Part model, mm, in its own coordinate system. Face numbers are marked on the shaded views. A direction names the side the tool comes from. Coordinates: 2 decimals unless noted, no trailing zeros. Loops run counter-clockwise (first coordinate to the right, second up) from the corner with the lowest first, then second, coordinate; pieces in that order, holes last. Notation, with made-up numbers: (49, 69) - (98, 69) arc R17 cw to (98, 78) - close; hole circle Ø1 at (49, -21.75). An arc over 180 degrees is marked (long way). Answer as CSV lines item,"result".
from build123d import *

# Parameters (mm, degrees)
SKETCH1_R           = 5
BASEHEAD_DEPTH      = 6
SKETCH2_R           = 3
BASEBODY_DEPTH      = 12
HEXAGONSOCKET_DEPTH = 3
TOPFILLET_R         = 0.75
CHAMFER1_SIZE       = 0.25
LPATTERN10_COUNT    = 18
LPATTERN10_PITCH    = 0.6498


with BuildPart() as part:
    # Sketch1 → BaseHead (new body)
    with BuildSketch(Plane(origin=(0, 0, 0), x_dir=(0, 0, -1), z_dir=(1, 0, 0))):
        Circle(SKETCH1_R)
    extrude(amount=BASEHEAD_DEPTH)

    # Sketch2 → BaseBody (add)
    with BuildSketch(Plane(origin=(6, 0, 0), x_dir=(0, 0, -1), z_dir=(1, 0, 0))):
        Circle(SKETCH2_R)
    extrude(amount=BASEBODY_DEPTH)

    # Sketch3 → HexagonSocket (cut)
    with BuildSketch(Plane(origin=(0, 0, 0), x_dir=(0, 0, -1), z_dir=(1, 0, 0))):
        Polygon((2.886751346, 0), (1.443375673, 2.5), (-1.443375673, 2.5), (-2.886751346, 0), (-1.443375673, -2.5), (1.443375673, -2.5), align=None)
    extrude(amount=HEXAGONSOCKET_DEPTH, mode=Mode.SUBTRACT)

    # Sketch4 → Cut-Revolve1 (revolve, cut)
    with BuildSketch(Plane(origin=(-4.19613823, 0.75, 0), x_dir=(-1, 0, 0), z_dir=(0, 0, 1))):
        Polygon((-7.19613823, 3.25), (-8.639513903, 0.75), (-7.19613823, 0.75), align=None)
    revolve(axis=Axis((0.838992387, 0, 0), (-1, 0, 0)), mode=Mode.SUBTRACT)

    # TopFillet
    topfillet_edges = [part.edges().sort_by_distance(p)[0] for p in [
        (0, 0, 5),
    ]]
    fillet(topfillet_edges, radius=TOPFILLET_R)

    # Chamfer1
    chamfer1_edges = [part.edges().sort_by_distance(p)[0] for p in [
        (18, 0, 3),
    ]]
    chamfer(chamfer1_edges, length=CHAMFER1_SIZE)

    # Sketch5 → Cut-Revolve10 (revolve, cut)
    with BuildSketch(Plane.XY):
        Polygon((17.75, 2.531047244), (18.02075, 3), (18.02075, 3.5415), (17.47925, 3.5415), (17.47925, 3), align=None)
    cut_revolve10 = revolve(axis=Axis((0, 0, 0), (1, 0, 0)), mode=Mode.SUBTRACT)

    # LPattern10: Cut-Revolve10 ×18
    with Locations(*[(-i * LPATTERN10_PITCH, 0, 0) for i in range(1, LPATTERN10_COUNT)]):
        add(cut_revolve10, mode=Mode.SUBTRACT)


solid = part.part
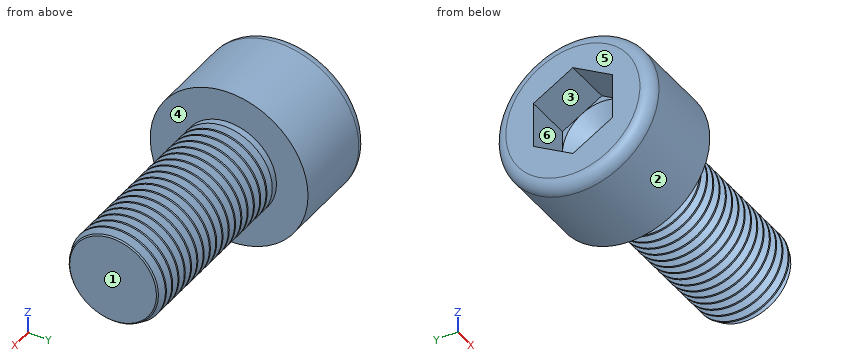
Q1. Saw through at A-A (x = 2.5). Give the cut face in (y, z).
Results:
outline,"circle Ø10 at (0, 0); hole (-2.5, -1.44) - (0, -2.89) - (2.5, -1.44) - (2.5, 1.44) - (0, 2.89) - (-2.5, 1.44) - close"
Q2. Wall check: L1, parallel to Y at x = 2.5, z = 0; L2, parallel to X at y = -2, z = 3.25; L3, parallel to Y at x = 2.75, z = 1.5. Give the ranges that are in metal, low to high.
Results:
L1,"y = -5 to -2.5, 2.5 to 5"
L2,"x = 0 to 6"
L3,"y = -4.77 to -2.4, 2.4 to 4.77"
Q3. Saw through at B-B (x = 5). Give the cut face in (y, z), then the cut area to 3 significant figures.
Results:
outline,"circle Ø10 at (0, 0)"
area,"78.5 mm^2"
Q4. Which spindle directions (+Z, -Z, +X, -X, +Y, -Y) get a long thin tool onto all of the face, cutting with end or side? Do the marked faces 4, 5 and 6. Say none if no direction does.
Results:
face 4,"+X"
face 5,"+Z, -Z, -X, +Y, -Y"
face 6,"-X"
Q5. Flat gauge pins, fed straight in: pin 1 (1 mm diameter, centred on x = 10, y = -3.5, fed in from -Z); pin 2 (1 mm diameter, centred on x = 6, y = -2, fed in from +Z); pin 3 (2 mm diameter, centred on x = 4.5, y = -2, fed in from +Z); pin 4 (2 mm diameter, centred on x = 9.5, y = 2, fed in from +Z). Where does each tip first touch, or does it go through?
Results:
pin 1,"passes through"
pin 2,"stops at z = 4.77"
pin 3,"stops at z = 4.9"
pin 4,"stops at z = 2.83"
Q6. Two-plate mould, pull along Y, no slides. Class the marked faces 1, 2 and 3: released by +Y, released by -Y, zero draft, split by the parting line, or undercut.
Results:
face 1,"zero draft"
face 2,"split by the parting line"
face 3,"undercut"
